Autodesk Inventor part; units mm, degrees
ref_plane "YZ Plane" through (0, 0, 0) normal (1, 0, 0) x (0, 1, 0)
ref_plane "XZ Plane" through (0, 0, 0) normal (0, 1, 0) x (-1, 0, 0)
ref_plane "XY Plane" through (0, 0, 0) normal (0, 0, 1) x (1, 0, 0)
sketch "Sketch1" plane through (0, 0, 0) normal (0, 1, 0) x (-1, 0, 0)
  line L0 (-6.5, 6.5) -> (6.5, 6.5)
  line L1 (6.5, 6.5) -> (6.5, -6.5)
  line L2 (6.5, -6.5) -> (-6.5, -6.5)
  line L3 (-6.5, -6.5) -> (-6.5, 6.5)
  line L4 (-6.5, 6.5) -> (6.5, -6.5) construction
  line L5 (6.5, 6.5) -> (-6.5, -6.5) construction
  circle A0 centre (10, 10) radius 2.375
  circle A1 centre (10, -10) radius 2.375
  circle A2 centre (-10, 10) radius 2.375
  circle A3 centre (-10, -10) radius 2.375
  line L6 (-14, 13) -> (14, 13)
  line L7 (14, 13) -> (14, -13)
  line L8 (14, -13) -> (-14, -13)
  line L9 (-14, -13) -> (-14, 13)
  line L10 (-14, 13) -> (14, -13) construction
  line L11 (14, 13) -> (-14, -13) construction
  line L12 (6.5, 6.5) -> (6.5, 13)
  line L13 (-6.5, 6.5) -> (-6.5, 13)
  line L14 (-6.5, -6.5) -> (-6.5, -13)
  line L15 (6.5, -6.5) -> (6.5, -13)
  point P0 (0, 0)
  dimension "d0" = 13
  dimension "d1" = 13
  dimension "d2" = 4.75
  dimension "d3" = 3.5
  dimension "d4" = 3.5
  dimension "d5" = 3.5
  dimension "d6" = 3.5
  dimension "d9" = 28
  dimension "d10" = 26
extrude "Extrusion1" add sketch "Sketch1" along normal blind 5 contours L3 L14 L8 L9 L6 L13 | L12 L6 L7 L8 L15 L1
extrude "Extrusion2" add sketch "Sketch1" along normal blind 2.5 contours L0 L1 L2 L3
properties part number "PCB_Housing_08_V4"
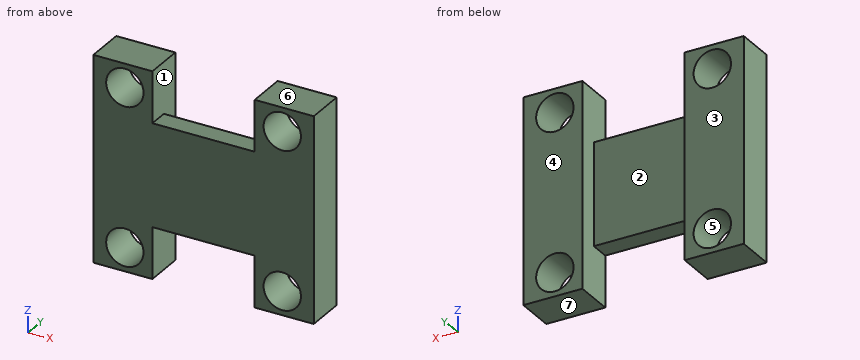
Check sheet for the modelled part. Datum: model origin and axes. Units: mm. Face numbers are marked on the shaded views. A direction names the side the tool comes from. Coordinates: 2 decimals unless noted, no trailing zeros. Order: outer loops, then holes, each group sorted by start corner. A loop starts at its lowest first (then second) coordinate and runs counter-clockwise, first axis right, second up. Notation, with made-up numbers: M -29,73 L -15,73 A22 cw -15,108 Z; hole C 9.25,73.25 d10. An arc over 180 degrees is marked long. Write each question's results on one line, items separated by ' | '. Start each with the question number.
1. Go/stop test with flat-tipped pins: P1, Ø3, axis at x = -1, y = 1, coming from the +Z side; P2, Ø1, axis at x = -5, z = -2, coming from the +Y side; P3, Ø3, axis at x = -1.5, y = 1.5, coming from the -Z side. Record where each tip stops, or that it passes through.
2. Cross-section at C-C on y = 4.6. Record the cut outline in (x, z) (3 decimals).
3. Mould release check, pull along Z, two halves, no side actions. Record for the marked faces 4, 5, 6 and 7: +Z half, -Z half, draft (parallel to the pull), parting line (faces both ways), or undercut.
4. Access from +Z, -Z, +X, -X, +Y, -Y to the whole of each face (thin tool, end or side, straight path). Record for the marked faces 1, 2 and 3.
5. Cross-section at D-D on y = 2.05. Record the cut outline in (x, z) (3 decimals).
6. Cross-section at A-A on z = -10. Record the cut outline in (x, y) (3 decimals).
7. Material ranges on probe 1 along Z at (x, y) = (10, 2.15) (3 decimals); probe 2 along X at (y, z) = (4.6, -1.25); probe 3 along Z at (x, y) = (9.5, 1.25), recorded low to high.
8. Cross-section at B-B on x = 10. Record the cut outline in (y, z) (3 decimals).
Checks:
1) P1: stops at z = 6.5 | P2: stops at y = 2.5 | P3: stops at z = -6.5
2) outline: M -14,-13 L -6.5,-13 L -6.5,13 L -14,13 Z; M 6.5,-13 L 14,-13 L 14,13 L 6.5,13 Z; hole C -10,-10 d4.75; hole C -10,10 d4.75; hole C 10,-10 d4.75; hole C 10,10 d4.75
3) face 4: draft | face 5: undercut | face 6: +Z half | face 7: -Z half
4) face 1: +Y | face 2: +Z, -Z, +Y | face 3: +Z, -Z, +X, -X, +Y
5) outline: M -14,-13 L -6.5,-13 L -6.5,-6.5 L 6.5,-6.5 L 6.5,-13 L 14,-13 L 14,13 L 6.5,13 L 6.5,6.5 L -6.5,6.5 L -6.5,13 L -14,13 Z; hole C -10,-10 d4.75; hole C -10,10 d4.75; hole C 10,-10 d4.75; hole C 10,10 d4.75
6) outline: M -14,0 L -12.375,0 L -12.375,5 L -14,5 Z; M -7.625,0 L -6.5,0 L -6.5,5 L -7.625,5 Z; M 6.5,0 L 7.625,0 L 7.625,5 L 6.5,5 Z; M 12.375,0 L 14,0 L 14,5 L 12.375,5 Z
7) probe 1: z = -13 to -12.375, -7.625 to 7.625, 12.375 to 13 | probe 2: x = -14 to -6.5, 6.5 to 14 | probe 3: z = -13 to -12.32, -7.68 to 7.68, 12.32 to 13
8) outline: M 0,-13 L 5,-13 L 5,-12.375 L 0,-12.375 Z; M 0,-7.625 L 5,-7.625 L 5,7.625 L 0,7.625 Z; M 0,12.375 L 5,12.375 L 5,13 L 0,13 Z
